Can you work these out from the model? Positions are in its coordinate system, mm. A direction names the side the tool comes from. Give positions to 0.01 mm unless a question says otherwise; leave off trailing zeros. Order: outer loops, then holes, each group sorted by start corner. A loop starts at its lowest first (then second) coordinate and runs counter-clockwise, first axis right, second up. Notation, with made-up numbers: (-37.5, 51.5) -> (17.5, 51.5) arc R13 cw to (17.5, 72.5) -> close; hole circle Ø2 at (75, 85.5). An arc over 180 degrees is marked (long way). Answer as CSV lines item,"result".
```python
from build123d import *

# Parameters (mm, degrees)
F0_R     = 20
F1_DEPTH = 5
F2_R     = 13.75
F3_DEPTH = 7
F5_SIZE  = 3
F4_R     = 11.25
F6_DEPTH = 7
F7_R     = 5
F8_DEPTH = 5


with BuildPart() as f1:
    # F0 (on Top) → F1 (new body)
    with BuildSketch(Plane.XY):
        Circle(F0_R)
    extrude(amount=F1_DEPTH)

    # F2 (on face) → F3 (join)
    with BuildSketch(Plane.XY.offset(5)):
        Circle(F2_R)
    extrude(amount=F3_DEPTH)

    # F5
    f5_edges = [f1.edges().sort_by_distance(p)[0] for p in [
        (-20, 0, 5),
    ]]
    chamfer(f5_edges, length=F5_SIZE)

    # F4 (on face) → F6 (cut)
    with BuildSketch(Plane.XY.offset(12)):
        Circle(F4_R)
    extrude(amount=-F6_DEPTH, mode=Mode.SUBTRACT)

    # F7 (on face) → F8 (cut, through all)
    with BuildSketch(Plane.XY.offset(5)):
        Circle(F7_R)
    extrude(amount=-F8_DEPTH, mode=Mode.SUBTRACT)


solid = f1.part
```
Item 1: Imagine slicing it at C-C, the plane z = 2.5. Please give me the cut outline in (x, y).
Numbers:
outline,"circle Ø39 at (0, 0); hole circle Ø10 at (0, 0)"
Item 2: Imagine slicing it at A-A, the plane y = 0. Please give me the cut outline in (x, z), then the cut area to 3 significant figures.
Numbers:
outline,"(-20, 0) -> (-5, 0) -> (-5, 5) -> (-11.25, 5) -> (-11.25, 12) -> (-13.75, 12) -> (-13.75, 5) -> (-17, 5) -> (-20, 2) -> close; (5, 0) -> (20, 0) -> (20, 2) -> (17, 5) -> (13.75, 5) -> (13.75, 12) -> (11.25, 12) -> (11.25, 5) -> (5, 5) -> close"
area,"176 mm²"
Item 3: Imagine slicing it at D-D, the plane z = 11. Please give me the cut outline in (x, y), then the cut area to 3 significant figures.
Numbers:
outline,"circle Ø27.5 at (0, 0); hole circle Ø22.5 at (0, 0)"
area,"196 mm²"
Item 4: For pin 1 (10 mm diameter, centred on x = 3.5, y = 3, fed in from +Z); pin 2 (3 mm diameter, centred on y = -5.5, z = 10.5, fed in from -X); pin 3 (3 mm diameter, centred on x = -13, z = 9.5, fed in from +Y), each with a flat end and sliding along its axis, tell me the tip position at first contact or that it passes through.
Numbers:
pin 1,"stops at z = 5"
pin 2,"stops at x = -13.16"
pin 3,"stops at y = 7.54"
Item 5: For faces 1 (the cylindrical face through (5.19, -9.98, 8.55)), 2 (the flat face through (4, -4, 0)), which set-ups out of +Z, -Z, +X, -X, +Y, -Y let a thin tool reach every point of the face, with its end or its side?
Numbers:
face 1,"+Z"
face 2,"-Z, +X, -X, +Y, -Y"
Item 6: Please list where these lines run through material, in increasing order: line 1 along Y through (x, z) = (0, 8.5); line 2 along Z through (x, y) = (5.5, 15); line 3 along Y through (x, z) = (-3, 5.25).
Numbers:
line 1,"y = -13.75 to -11.25, 11.25 to 13.75"
line 2,"z = 0 to 5"
line 3,"y = -13.42 to -10.84, 10.84 to 13.42"
